```python
from build123d import *

# Parameters (mm, degrees)
SM_BASE_FLANGE_1_DEPTH = 300


# Sheet-metal steps are written as plain solids
with BuildPart() as part:
    # Sketch 1 → 基体-法兰1 (new body)
    with BuildSketch(Plane.XY):
        with BuildLine():
            Line((-200, 300), (-0.1, 300))
            ThreePointArc((-0.1, 300), (-0.029289322, 299.970710678), (0, 299.9))
            Line((0, 299.9), (0, 2.1))
            ThreePointArc((0, 2.1), (0.61507576, 0.61507576), (2.1, 0))
            Line((2.1, 0), (499.130151519, 0))
            ThreePointArc((499.130151519, 0), (499.933786727, 0.159852982), (500.61507576, 0.61507576))
            Line((500.61507576, 0.61507576), (804.05591591, 304.05591591))
            ThreePointArc((804.05591591, 304.05591591), (992.143758514, 318.593525064), (1035.4112588, 134.973531505))
            Line((1035.4112588, 134.973531505), (1037.188153416, 134.055574248))
            ThreePointArc((1037.188153416, 134.055574248), (993.323860022, 320.208257373), (802.641702348, 305.470129473))
            Line((802.641702348, 305.470129473), (499.200862197, 2.029289322))
            ThreePointArc((499.200862197, 2.029289322), (499.168419862, 2.007612047), (499.130151519, 2))
            Line((499.130151519, 2), (2.1, 2))
            ThreePointArc((2.1, 2), (2.029289322, 2.029289322), (2, 2.1))
            Line((2, 2.1), (2, 299.9))
            ThreePointArc((2, 299.9), (1.38492424, 301.384924241), (-0.100000001, 302))
            Line((-0.1, 302), (-200, 302))
            Line((-200, 302), (-200, 300))
        make_face()
    extrude(amount=-SM_BASE_FLANGE_1_DEPTH)


solid = part.part
```
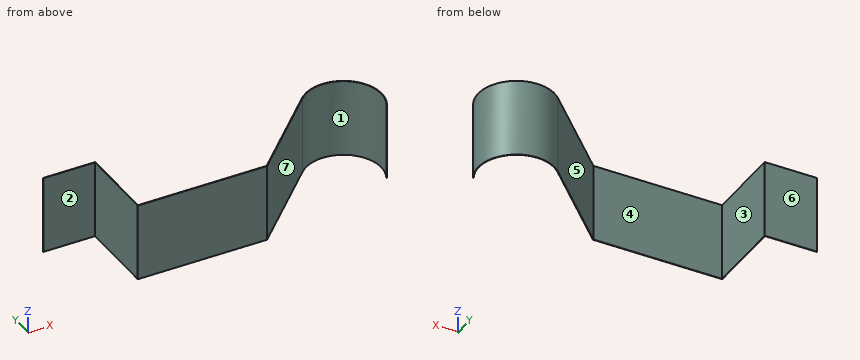
The listing builds one solid part. Answer for the finished solid, in the listing's coordinates (mm). Face numbers are marked on the shaded views. A direction names the side the tool comes from. Give positions to 0.01 mm unless a question says otherwise; leave off trailing zeros. Order: outer loops, then holes, each group sorted by start corner. A loop starts at its lowest first (then second) coordinate and runs counter-clockwise, first axis right, second up.
1) Find section A-A on y = 240. Write down the section's boundary in (x, z), then the cut area to 3 significant figures.
Reported:
outline: (0, -300) - (2, -300) - (2, 0) - (0, 0) - close; (737.17, -300) - (740, -300) - (740, 0) - (737.17, 0) - close; (1046.39, -300) - (1048.46, -300) - (1048.46, 0) - (1046.39, 0) - close
area: 2,070 mm2
2) Determine the mould class of the marked faces 1, 2, 3 and 4 for opening direction Y: pulls with the +Y half, pulls with the -Y half, needs draft (parallel to the pull), parting line crosses it, or undercut.
Reported:
face 1: undercut
face 2: pulls with the -Y half
face 3: needs draft
face 4: pulls with the +Y half
3) Find section D-D on y = 152.5. Write down the section's boundary in (x, z).
Reported:
outline: (0, -300) - (2, -300) - (2, 0) - (0, 0) - close; (649.67, -300) - (652.5, -300) - (652.5, 0) - (649.67, 0) - close; (1043.05, -300) - (1045.17, -300) - (1045.17, 0) - (1043.05, 0) - close
4) Find section C-C on y = 101. Write down the section's boundary in (x, z), then the cut area to 3 significant figures.
Reported:
outline: (0, -300) - (2, -300) - (2, 0) - (0, 0) - close; (598.17, -300) - (601, -300) - (601, 0) - (598.17, 0) - close
area: 1,450 mm2
5) Given P1, Ø6, axis at y = 146, z = -57.5, coming from the -X side; P2, Ø3, axis at y = 160, z = -102.5, coming from the +X side; P3, Ø1.5, axis at x = 552, z = -131, coming from the -Y side, each flat-ended and moving along its own axis, determine where each tip first touches the part or whether it passes through.
Reported:
P1: stops at x = 0
P2: stops at x = 1048.03
P3: stops at y = 51.25
6) Consider line 1 along X through (y, z) = (279, -276.5); line 2 along X through (y, z) = (284, -28.5); line 3 along Y through (x, z) = (299.5, -186). Determine where each line is inside the solid, lowest interval first.
Reported:
line 1: x = 0 to 2, 776.17 to 779, 1029.15 to 1031.51
line 2: x = 0 to 2, 781.17 to 784, 1025.85 to 1028.27
line 3: y = 0 to 2
7) For the marked faces 5, 6 and 7, determine the directions among +Z, -Z, +X, -X, +Y, -Y from which every point of the face is accessible in a straight line to the end or side of a thin tool.
Reported:
face 5: +Z, -Z, +Y
face 6: +Z, -Z, -X, +Y
face 7: +Z, -Z, -Y
8) Find section B-B on z = -92. Write down the section's boundary in (x, y), then the cut area to 3 significant figures.
Reported:
outline: (-200, 300) - (-0.1, 300) arc R0.1 cw to (0, 299.9) - (0, 2.1) arc R2.1 ccw to (2.1, 0) - (499.13, 0) arc R2.1 ccw to (500.62, 0.62) - (804.06, 304.06) arc R145 cw to (1035.41, 134.97) - (1037.19, 134.06) arc R147 ccw to (802.64, 305.47) - (499.2, 2.03) arc R0.1 cw to (499.13, 2) - (2.1, 2) arc R0.1 cw to (2, 2.1) - (2, 299.9) arc R2.1 ccw to (-0.1, 302) - (-200, 302) - close
area: 3,680 mm2
